Model file for the job. Use its own axes, mm. A direction names the side the tool comes from. Give positions to 0.01 mm unless a question says otherwise; leave off trailing zeros. Write each loop counter-clockwise with the first axis right and the second up, starting at its lowest first coordinate (ties: lowest second). Pieces come first, ordered by that corner, then holes. Notation, with made-up numbers: (31.5, 53.25) - (69.5, 53.25) arc R15 cw to (69.5, 66.25) - close; hole circle Ø8 at (10, -24.5). An arc over 180 degrees is marked (long way). One line per item, written item: value. Start each with the question number.
(1) Probe L1, parallel to Y at x = -33.5, z = 11.5; L2, parallel to Z at x = 33, y = 0; L3, parallel to Y at x = -42, z = 0. List the from-to ranges inside material, lowest first.
(2) Cut at A-A, the plane z = 11.5. List the corners of the cut face in (x, y).
(3) Drop flat-ended pins along their axis: P1, Ø3.5, axis at y = 32.5, z = -3, coming from the -X side; P2, Ø5.5, axis at y = -6.5, z = 11.5, coming from the +X side; P3, Ø4, axis at y = -18, z = 3.5, coming from the +X side. Give the stop position or say it passes through.
(4) Mould opens along X. For faces 5 (the face through (-31, 0, -15)), 6 (the face through (-45.5, -4.1, -1.5)), 7 (the face through (0.536, -30.495, -0.21)) say: pulls with the +X half, pulls with the -X half, needs draft (parallel to the pull), parting line crosses it, or undercut.
(5) Cut at B-B, the plane y = 15. List the corners of the cut face in (x, z).
(6) Cut at C-C, the plane x = -16. List the corners of the cut face in (y, z).
(7) 3-axis set-ups, long thin cutter, end or side, ignore diameter. For faces 1 (the face through (-35, 10, 0)), 2 (the face through (-18.72, 24.08, -0.21)), 3 (the face through (35.15, 3.4, 3.4)), 4 (the face through (1.5, 32, 0)): which of +Z, -Z, +X, -X, +Y, -Y reach the whole face in a straight line?
(8) Cut at D-D, the plane x = -30. List the corners of the cut face in (y, z).
Autodesk Inventor part; units mm, degrees
ref_plane "Work Plane2" through (-33.5, 0, 0) normal (1, 0, 0) x (0, 1, 0)
ref_plane "XZ Plane" through (0, 0, 0) normal (0, 1, 0) x (-1, 0, 0)
ref_plane "XY Plane" through (0, 0, 0) normal (0, 0, 1) x (1, 0, 0)
sketch "Sketch1" plane through (0, 0, 0) normal (0, 0, 1) x (1, 0, 0)
  circle A0 centre (0, 0) radius 30.5
  circle A1 centre (0, 0) radius 33.5
  dimension "d0" = 61
  dimension "d1" = 67
extrude "Extrusion1" add sketch "Sketch1" along normal mid plane 30
ref_plane "Work Plane2" through (-33.5, 0, 0) normal (1, 0, 0) x (0, 1, 0)
ref_plane "Work Plane1" through (33.5, 0, 0) normal (1, 0, 0) x (0, 1, 0)
sketch "Sketch3" plane through (33.5, 0, 0) normal (1, 0, 0) x (0, 1, 0)
  line L0 (-30.5, 15) -> (30.5, 15)
  line L1 (-10, -15) -> (10, -15)
  line L2 (10, -15) -> (10, 15)
  line L3 (10, 15) -> (-10, 15)
  line L4 (-10, 15) -> (-10, -15)
  line L5 (-10, -15) -> (10, 15) construction
  line L6 (10, -15) -> (-10, 15) construction
  point P0 (0, 0)
  dimension "d20" = 20
extrude "Extrusion2" add sketch "Sketch3" along normal blind 4 and the other way blind 4.5
sketch "Sketch4" plane through (-33.5, 0, 0) normal (1, 0, 0) x (0, 1, 0)
  line L0 (30.5, -15) -> (-30.5, -15)
  line L1 (10, 15) -> (-10, 15)
  line L2 (-10, 15) -> (-10, -15)
  line L3 (-10, -15) -> (10, -15)
  line L4 (10, -15) -> (10, 15)
  line L5 (10, 15) -> (-10, -15) construction
  line L6 (-10, 15) -> (10, -15) construction
  point P0 (0, 0)
  dimension "d25" = 20
extrude "Extrusion3" add sketch "Sketch4" along normal blind 4.5 and the other way blind 4
sketch "Sketch5" plane through (33.5, 0, 0) normal (1, 0, 0) x (0, 1, 0)
  circle A0 centre (0, 0) radius 3.5
  circle A1 centre (0, 0) radius 6.25
  dimension "d30" = 7
  dimension "d31" = 12.5
extrude "Extrusion4" add sketch "Sketch5" along normal blind 12
sketch "Sketch6" plane through (-37.5, 0, 0) normal (-1, 0, 0) x (0, 0, 1)
  circle A0 centre (0, 0) radius 3.5
  circle A1 centre (0, 0) radius 6.25
  dimension "d35" = 7
  dimension "d36" = 12.5
extrude "Extrusion5" add sketch "Sketch6" along normal blind 8
sketch "Sketch8" plane through (-29, 0, 0) normal (1, 0, 0) x (0, 0, -1)
  point P0 (0, 0)
  point P1 (0, 0)
hole "Hole3" at (-29, 0, 0) direction (-1, 0, 0) diameter 8.4 depth 16.5 counterbore diameter 16 counterbore depth 6.15
sketch "Sketch9" plane through (29, 0, 0) normal (-1, 0, 0) x (0, 0, 1)
  point P0 (0, 0)
  point P1 (0, 0)
hole "Hole4" at (29, 0, 0) direction (1, 0, 0) diameter 8.4 depth 16.5 counterbore diameter 16 counterbore depth 6.15
sketch "Sketch10" plane through (-37.5, 0, 0) normal (-1, 0, 0) x (0, 0, 1)
  line L0 (-15, 10) -> (-15, -10)
  line L1 (15, -10) -> (15, 10)
  line L2 (-15, -10) -> (15, -10)
  point P0 (0, 0)
  point P1 (11.5, -6.5)
  point P2 (-11.5, -6.5)
  dimension "d58" = 3.5
  dimension "d59" = 3.5
  dimension "d60" = 3.5
hole "Hole5" at (-37.5, -6.5, 11.5) at (-37.5, -6.5, -11.5) direction (1, 0, 0) diameter 4.134 depth 75
sketch "Sketch11" plane through (0, 0, 15) normal (0, 0, 1) x (1, 0, 0)
  line L0 (-1.5, 37.1959) -> (1.5, 37.1959)
  line L1 (1.5, 37.1959) -> (1.5, 23.2844)
  line L2 (1.5, 23.2844) -> (-1.5, 23.2844)
  line L3 (-1.5, 23.2844) -> (-1.5, 37.1959)
  point P0 (0, 0)
  dimension "d68" = 1.5
  dimension "d69" = 1.5
extrude "Extrusion7" cut sketch "Sketch11" against normal through all
equation "\"d25\" = d20"
properties part number "Soporte_PVC_Balancin"
Answers follow:
1. L1: y = -10 to -8.57, -4.43 to 10
1. L2: z = -15 to -8, 8 to 15
1. L3: y = -6.25 to -4.2, 4.2 to 6.25
2. outline: (-37.5, -10) - (-31.97, -10) arc R33.5 ccw to (31.97, -10) - (37.5, -10) - (37.5, -8.57) - (29, -8.57) - (29, -9.45) arc R30.5 cw to (-29, -9.45) - (-29, -8.57) - (-37.5, -8.57) - close; (-37.5, -4.43) - (-29, -4.43) - (-29, 9.45) arc R30.5 cw to (-1.5, 30.46) - (-1.5, 33.47) arc R33.5 ccw to (-31.97, 10) - (-37.5, 10) - close; (1.5, 30.46) arc R30.5 cw to (29, 9.45) - (29, -4.43) - (37.5, -4.43) - (37.5, 10) - (31.97, 10) arc R33.5 ccw to (1.5, 33.47) - close
3. P1: stops at x = -13.29
3. P2: stops at x = 37.5
3. P3: stops at x = 29.43
4. face 5: needs draft
4. face 6: pulls with the -X half
4. face 7: undercut
5. outline: (-29.95, -15) - (-26.56, -15) - (-26.56, 15) - (-29.95, 15) - close; (26.56, -15) - (29.95, -15) - (29.95, 15) - (26.56, 15) - close
6. outline: (-29.43, -15) - (-25.97, -15) - (-25.97, 15) - (-29.43, 15) - close; (25.97, -15) - (29.43, -15) - (29.43, 15) - (25.97, 15) - close
7. face 1: +Z, -Z, -X, +Y
7. face 2: +Z, -Z
7. face 3: none
7. face 4: +Z, -Z, +Y
8. outline: (-14.91, -15) - (14.91, -15) - (14.91, 15) - (-14.91, 15) - close; hole circle Ø4.13 at (-6.5, -11.5); hole circle Ø4.13 at (-6.5, 11.5); hole circle Ø16 at (0, 0)
